Design review of the part built by this model. Coordinates are the model's own, in mm. A direction names the side the tool comes from. Round coordinates to 2 decimals unless told otherwise and drop trailing zeros. Order: outer loops, then holes, each group sorted by start corner. A loop starts at its lowest first (then second) coordinate and runs counter-clockwise, first axis right, second up.
from build123d import *

# Parameters (mm, degrees)
SKETCH1_W           = 412
SKETCH1_H           = 412
SKETCH1_W_2         = 400
SKETCH1_H_2         = 400
EXTRUDE_THIN1_DEPTH = 200
SKETCH5_W           = 462
SKETCH5_H           = 462
SKETCH5_W_2         = 412
SKETCH5_H_2         = 412
EXTRUDE_THIN2_DEPTH = 12
SKETCH6_R           = 2.15
CUT_EXTRUDE1_DEPTH  = 380.944732823


with BuildPart() as part:
    # Sketch1 → Extrude-Thin1 (new body)
    with BuildSketch(Plane(origin=(0, 0, 0), x_dir=(0, 0, -1), z_dir=(1, 0, 0))):
        Rectangle(SKETCH1_W, SKETCH1_H)
        Rectangle(SKETCH1_W_2, SKETCH1_H_2, mode=Mode.SUBTRACT)
    extrude(amount=EXTRUDE_THIN1_DEPTH)

    # Sketch5 → Extrude-Thin2 (add)
    with BuildSketch(Plane(origin=(194, 0, 0), x_dir=(0, 0, -1), z_dir=(1, 0, 0))):
        Rectangle(SKETCH5_W, SKETCH5_H)
        Rectangle(SKETCH5_W_2, SKETCH5_H_2, mode=Mode.SUBTRACT)
    extrude(amount=-EXTRUDE_THIN2_DEPTH)

    # Sketch6 → Cut-Extrude1 (cut, through all)
    with BuildSketch(Plane(origin=(194, 0, 0), x_dir=(0, 0, -1), z_dir=(1, 0, 0))):
        with BuildLine():
            ThreePointArc((-216.35, 218.5), (-217.67723062, 220.486340995), (-220.02027958, 220.02027958))
            Line((-220.02027958, 220.02027958), (-216.97972042, 216.97972042))
            ThreePointArc((-216.97972042, 216.97972042), (-216.513659005, 217.67723062), (-216.35, 218.5))
        make_face()
        with BuildLine():
            Line((-216.97972042, 216.97972042), (-220.02027958, 220.02027958))
            ThreePointArc((-220.02027958, 220.02027958), (-220.02027958, 216.97972042), (-216.97972042, 216.97972042))
        make_face()
        with Locations((-72.83, 218.5)):
            Circle(SKETCH6_R)
        with Locations((72.84, 218.5)):
            Circle(SKETCH6_R)
        with Locations((-218.5, -72.84)):
            Circle(SKETCH6_R)
        with Locations((-72.83, -218.5)):
            Circle(SKETCH6_R)
        with Locations((72.84, -218.5)):
            Circle(SKETCH6_R)
        with Locations((218.5, -72.84)):
            Circle(SKETCH6_R)
        with Locations((-218.5, 72.83)):
            Circle(SKETCH6_R)
        with Locations((-218.5, -218.5)):
            Circle(SKETCH6_R)
        with Locations((218.5, -218.5)):
            Circle(SKETCH6_R)
        with Locations((218.5, 72.83)):
            Circle(SKETCH6_R)
        with Locations((218.5, 218.5)):
            Circle(SKETCH6_R)
    extrude(amount=-CUT_EXTRUDE1_DEPTH, mode=Mode.SUBTRACT)


solid = part.part
1) Take a section at C-C on x = 71.5. Give the boundary of the cut face in (y, z), plus the area to 3 significant figures.
Results:
outline: (-206, -206) - (206, -206) - (206, 206) - (-206, 206) - close; hole (-200, -200) - (200, -200) - (200, 200) - (-200, 200) - close
area: 9,740 mm2
2) For faces 1 (the face through (90, -3, 206)), 2 (the face through (99, -200, 3)), 3 (the face through (90, -206, 3)), list the 3-axis set-ups (+Z, -Z, +X, -X, +Y, -Y) from which the entire face can be reached by the end or side of a thin tool; tool diameter is ignored.
Results:
face 1: +Z, -X, +Y, -Y
face 2: +X, -X
face 3: +Z, -Z, -X, -Y
3) To check wall thickness, follow line 1 along Z through (x, y) = (186, -218); line 2 along Y through (x, z) = (191.5, 218.5); line 3 along Y through (x, z) = (135.5, -125). State the ranges of each line that lie inside material, in increasing order.
Results:
line 1: z = -231 to -220.59, -216.41 to -74.93, -70.75 to 70.74, 74.92 to 216.41, 220.59 to 231
line 2: y = -231 to -220.65, -216.35 to -74.99, -70.69 to 70.68, 74.98 to 216.35, 220.65 to 231
line 3: y = -206 to -200, 200 to 206
4) The part is to be moulded in two halves that separate along Y. For faces 4 (the face through (188, 231, 3)), 5 (the face through (182, 35.3, 206.4)), 6 (the face through (99, -3, 200)), say which applies: released by +Y, released by -Y, zero draft, split by the parting line, or undercut.
Results:
face 4: released by +Y
face 5: zero draft
face 6: undercut
5) Clearance check with flat-ended pins moving along their axes: P1, Ø3.5, axis at y = 72.83, z = -218.5, coming from the -X side; P2, Ø8, axis at x = 156.5, z = 141, coming from the -Y side; P3, Ø1.8, axis at x = 198.5, y = 41, coming from the -Z side; P4, Ø1, axis at x = 65.5, z = -128, coming from the +Y side. State where each tip first meets the part, or that it passes through.
Results:
P1: passes through
P2: stops at y = -206
P3: stops at z = -206
P4: stops at y = 206
6) Take a section at A-A on y = 8. Give the boundary of the cut face in (x, z).
Results:
outline: (0, -206) - (182, -206) - (182, -231) - (194, -231) - (194, -206) - (200, -206) - (200, -200) - (0, -200) - close; (0, 200) - (200, 200) - (200, 206) - (194, 206) - (194, 231) - (182, 231) - (182, 206) - (0, 206) - close
